The listing builds one solid part. Answer for the finished solid, in the listing's coordinates (mm). A direction names the side the tool comes from. Coordinates: 2 decimals unless noted, no trailing zeros. Write each loop counter-clockwise with the first axis right and the second up, starting at its lowest first coordinate (ties: lowest second). Pieces come first, ordered by that corner, then holes.
(1) For a pull along Z with two mould halves and no side action, classify faces 1 (the flat face through (3, -31, 10)), 2 (the flat face through (-48.7, -23.1, 55)), 3 (the flat face through (29, -5, 32)), 4 (the flat face through (3, -26, 15)) as +Z half, -Z half, draft (parallel to the pull), parting line (faces both ways), or undercut.
(2) The part is cut by section D-D on x = -52. Determine the outline of the cut face in (y, z), plus the area to 3 significant figures.
(3) The part is cut by section C-C on y = -7. Determine the outline of the cut face in (x, z).
(4) The part is cut by section A-A on y = -23. Determine the outline of the cut face in (x, z).
(5) Given P1, Ø5, axis at x = -66.5, y = -24.5, coming from the -Z side; P2, Ø2, axis at y = -20.5, z = 11, coming from the +X side; P3, Ø10, axis at x = 34, y = -15.5, coming from the +Z side; P4, Ø3.5, axis at x = -68, y = -7, coming from the +Z side, each flat-ended and moving along its own axis, determine where each tip first touches the part or whether it passes through.
(6) The part is cut by section B-B on z = 9. Determine the outline of the cut face in (x, y), plus the area to 3 significant figures.
(7) Straight lines are drawn through the part: line 1 (X direction, y = -7, z = 53.7); line 2 (Y direction, x = -68, z = 57); line 3 (Y direction, x = -68, z = 53.95). For each, find the intervals that lie inside material, in ascending order.
(8) Which of the six approach directions +Z, -Z, +X, -X, +Y, -Y give full straight-line access (tool end or side, diameter ignored) to faces 5 (the flat face through (-48.7, -7.1, 55)), 6 (the flat face through (-35, -30, 56)), 7 (the flat face through (-37, -15, 53))?
Autodesk Fusion 360 part; units mm, degrees
sketch "Sketch1" plane through (0, 0, 0) normal (0, 0, 1) x (1, 0, 0)
  line L0 (0, 0) -> (52, 0)
  line L1 (52, 0) -> (52, -54)
  line L2 (52, -54) -> (0, -54)
  line L3 (0, -54) -> (0, 0)
  dimension "d1" = 52
  dimension "d2" = 54
extrude "Extrude1" add sketch "Sketch1" along normal blind 58
sketch "Sketch2" plane through (52, 0, 0) normal (1, 0, 0) x (0, 1, 0)
  line L0 (-54, 0) -> (0, 0)
  line L1 (0, 0) -> (0, 58)
  line L2 (0, 58) -> (-54, 58)
  line L3 (-54, 58) -> (-54, 0)
  line L4 (-5, 5) -> (-49, 5)
  line L5 (-49, 5) -> (-49, 53)
  line L6 (-49, 53) -> (-5, 53)
  line L7 (-5, 53) -> (-5, 5)
  dimension "d5" = 44
  dimension "d6" = 48
extrude "Extrude2" cut sketch "Sketch2" against normal blind 47 contours L4 L5 L6 L7
sketch "Sketch3" plane through (0, 0, 58) normal (0, 0, 1) x (-1, 0, 0)
  line L0 (0, 54) -> (-52, 54)
  line L1 (-52, 54) -> (-52, 0)
  line L2 (-52, 0) -> (0, 0)
  line L3 (0, 0) -> (0, 54)
  line L4 (-52, 5) -> (-5, 5)
  line L5 (-5, 5) -> (-5, 49)
  line L6 (-5, 49) -> (-52, 49)
  line L7 (-52, 49) -> (-52, 5)
  dimension "d9" = 47
  dimension "d10" = 44
extrude "Extrude3" cut sketch "Sketch3" against normal blind 6 contours L1 L4 L5 L6 L7
sketch "Sketch4" plane through (0, 0, 58) normal (0, 0, 1) x (-1, 0, 0)
  line L0 (-5, 5) -> (-52, 5)
  line L1 (-52, 5) -> (-52, 0)
  line L2 (-52, 0) -> (0, 0)
  line L3 (0, 0) -> (0, 54)
  line L4 (0, 54) -> (-52, 54)
  line L5 (0, 0) -> (75, 0)
  line L6 (75, 0) -> (75, 30)
  line L7 (75, 30) -> (0, 30)
  line L8 (0, 30) -> (0, 0)
  line L9 (-52, 54) -> (-52, 49)
  line L10 (-52, 49) -> (-5, 49)
  line L11 (-5, 49) -> (-5, 5)
  dimension "d13" = 75
  dimension "d14" = 30
extrude "Extrude4" add sketch "Sketch4" against normal blind 5 contours L3 L5 L6 L7 L8
sketch "Sketch5" plane through (0, 0, 58) normal (0, 0, 1) x (-1, 0, 0)
  line L0 (-5, 5) -> (-52, 5)
  line L1 (-52, 5) -> (-52, 0)
  line L2 (-52, 0) -> (75, 0)
  line L3 (75, 0) -> (75, 30)
  line L4 (75, 30) -> (0, 30)
  circle A0 centre (68, 7) radius 3
  circle A1 centre (68, 23) radius 3
  circle A2 centre (52, 7) radius 3
  circle A3 centre (52, 23) radius 3
  line L5 (0, 30) -> (0, 54)
  line L6 (0, 54) -> (-52, 54)
  line L7 (-52, 54) -> (-52, 49)
  line L8 (-52, 49) -> (-5, 49)
  line L9 (-5, 49) -> (-5, 5)
  dimension "d17" = 6
  dimension "d18" = 6
  dimension "d19" = 6
  dimension "d20" = 6
extrude "Extrude5" cut sketch "Sketch5" against normal blind 5 contours A0 | A1 | A2 | A3
sketch "Sketch6" plane through (0, 0, 53) normal (0, 0, -1) x (1, 0, 0)
  circle A0 centre (-68, 23) radius 3
  circle A1 centre (-68, 7) radius 3
  circle A2 centre (-52, 23) radius 3
  circle A3 centre (-52, 7) radius 3
  line L0 (0, 0) -> (0, 30)
  line L1 (0, 30) -> (-75, 30)
  line L2 (-75, 30) -> (-75, 0)
  line L3 (-75, 0) -> (0, 0)
  circle A4 centre (-68, 23) radius 5
  circle A5 centre (-52, 23) radius 5
  circle A6 centre (-68, 7) radius 5
  circle A7 centre (-52, 7) radius 5
  dimension "d23" = 10
  dimension "d24" = 10
  dimension "d25" = 10
  dimension "d26" = 10
extrude "Extrude6" cut sketch "Sketch6" against normal blind 2 contours A4 | A5 | A6 | A7
fillet "Fillet1" radius 5 2 edges at (-75, -30, 55.5) (-75, 0, 55.5)
sketch "Sketch7" plane through (5, 0, 0) normal (1, 0, 0) x (0, 1, 0)
  line L0 (-49, 58) -> (-49, 5)
  line L1 (-49, 5) -> (-5, 5)
  line L2 (-5, 5) -> (-5, 58)
  line L3 (-5, 58) -> (-49, 58)
  line L4 (-31, 5) -> (-21, 5)
  line L5 (-21, 5) -> (-21, 15)
  line L6 (-21, 15) -> (-31, 15)
  line L7 (-31, 15) -> (-31, 5)
  dimension "d31" = 10
  dimension "d32" = 10
extrude "Extrude7" cut sketch "Sketch7" against normal blind 15 contours L1 L4 L5 L6 L7
Model answer:
1. face 1: undercut
1. face 2: -Z half
1. face 3: draft
1. face 4: undercut
2. outline: (-30, 53) - (-28, 53) - (-28, 55) - (-26, 55) - (-26, 58) - (-30, 58) - close; (-20, 55) - (-18, 55) - (-18, 53) - (-12, 53) - (-12, 55) - (-10, 55) - (-10, 58) - (-20, 58) - close; (-4, 55) - (-2, 55) - (-2, 53) - (0, 53) - (0, 58) - (-4, 58) - close
2. area: 74.0 mm2
3. outline: (-75, 53) - (-73, 53) - (-73, 55) - (-71, 55) - (-71, 58) - (-75, 58) - close; (-65, 55) - (-63, 55) - (-63, 53) - (-57, 53) - (-57, 55) - (-55, 55) - (-55, 58) - (-65, 58) - close; (-49, 55) - (-47, 55) - (-47, 53) - (0, 53) - (0, 0) - (52, 0) - (52, 5) - (5, 5) - (5, 58) - (-49, 58) - close
4. outline: (-75, 53) - (-73, 53) - (-73, 55) - (-71, 55) - (-71, 58) - (-75, 58) - close; (-65, 55) - (-63, 55) - (-63, 53) - (-57, 53) - (-57, 55) - (-55, 55) - (-55, 58) - (-65, 58) - close; (-49, 55) - (-47, 55) - (-47, 53) - (0, 53) - (0, 15) - (5, 15) - (5, 58) - (-49, 58) - close; (0, 0) - (52, 0) - (52, 5) - (0, 5) - close
5. P1: stops at z = 55
5. P2: stops at x = 5
5. P3: stops at z = 5
5. P4: passes through
6. outline: (0, -54) - (52, -54) - (52, -49) - (5, -49) - (5, -31) - (0, -31) - close; (0, -21) - (5, -21) - (5, -5) - (52, -5) - (52, 0) - (0, 0) - close
6. area: 690 mm2
7. line 1: x = -75 to -73, -63 to -57, -47 to 5
7. line 2: y = -30 to -26, -20 to -10, -4 to 0
7. line 3: y = -30 to -28, -18 to -12, -2 to 0
8. face 5: -Z
8. face 6: +Z, -Z, -X, -Y
8. face 7: -Z, -X, +Y, -Y
